Part print with two shaded views. Sizes in mm from the minimum x, y, z corner. A direction names the side the tool comes from. Round coordinates to 2 decimals unless told otherwise and drop trailing zeros. Write each loop counter-clockwise with the first axis right and the second up, starting at its lowest first coordinate (ties: lowest second). Pieces come first, ordered by that corner, then holes. Notation, with made-up numbers: (-31, -4.75) - (27, -4.75) arc R17 cw to (27, 4.25) - close; hole circle Ø7 at (-34, 63). An arc over 180 degrees is marked (long way). Answer as a JSON object with one key per item and string values. Group by question number.
Item 1: Flat gauge pin, fed straight in: pin 1 (1.5 mm diameter, centred on x = 41, z = 7.5, fed in from +Y). Where does the tip first touch, or does it go through?
Item 2: Slice it at B-B, the plane x = 22.86. List the corners of the cut face in (y, z).
Item 3: Two-plate mould, pull along X, no slides. Class the marked faces 1, 2 and 3: +X half, -X half, draft (parallel to the pull), parting line (faces both ways), or undercut.
Item 4: Which spindle directions (+Z, -Z, +X, -X, +Y, -Y) get a long thin tool onto all of the face, cutting with end or side? Do the marked faces 4 and 5. Say none if no direction does.
Item 5: Slice it at A-A, the plane z = 8.89. List the corners of the cut face in (x, y).
Item 6: Slice it at C-C, the plane y = 26. List the corners of the cut face in (x, z).
Item 7: Probe line 1 (X direction, y = 2.4, z = 8.89); line 2 (Z direction, x = 25, y = 19); line 3 (X direction, y = 35, z = 9.5). List the from-to ranges inside material, lowest first. Write a range as from..to.
Item 8: Slice it at D-D, the plane x = 10.5. List the corners of the cut face in (y, z).
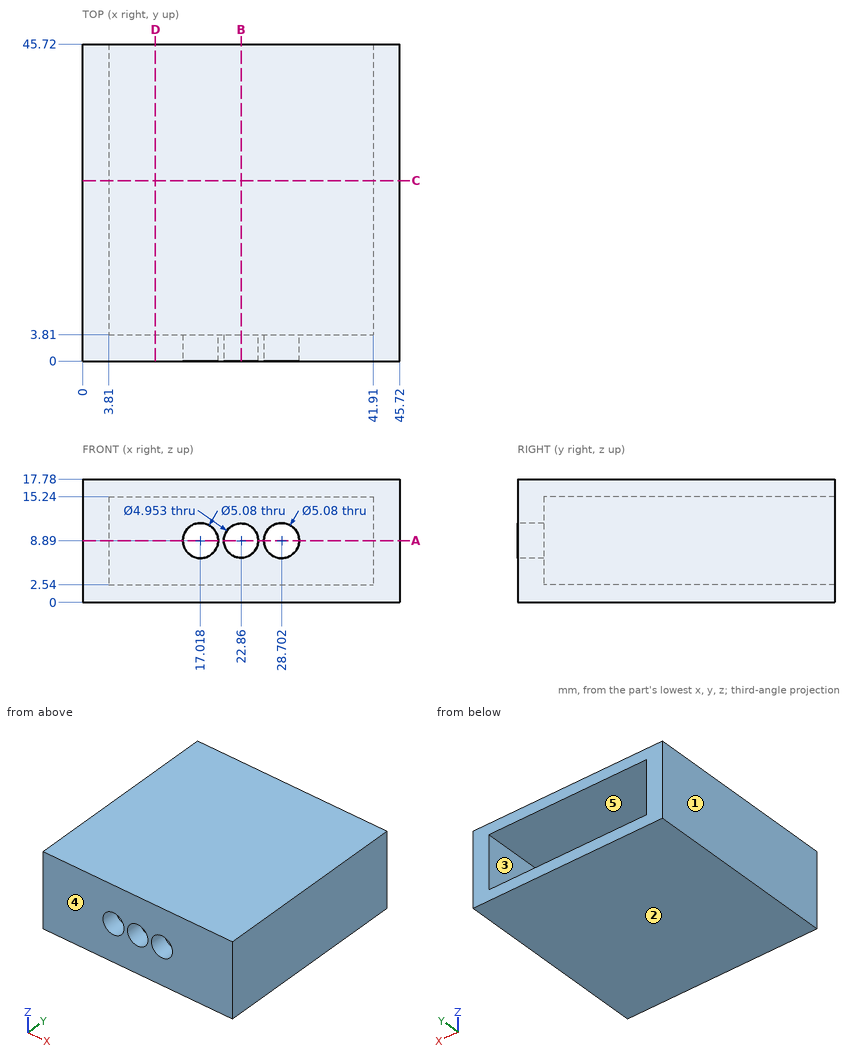
Geometry says:
{
 "1": {"pin 1": "stops at y = 3.81"},
 "2": {"outline": "(0, 0) - (45.72, 0) - (45.72, 2.54) - (3.81, 2.54) - (3.81, 6.41) - (0, 6.41) - close; (0, 11.37) - (3.81, 11.37) - (3.81, 15.24) - (45.72, 15.24) - (45.72, 17.78) - (0, 17.78) - close"},
 "3": {"face 1": "-X half", "face 2": "draft", "face 3": "undercut"},
 "4": {"face 4": "+Z, -Z, +X, -X, -Y", "face 5": "+Y"},
 "5": {"outline": "(0, 0) - (14.48, 0) - (14.48, 3.81) - (3.81, 3.81) - (3.81, 45.72) - (0, 45.72) - close; (19.56, 0) - (20.38, 0) - (20.38, 3.81) - (19.56, 3.81) - close; (25.34, 0) - (26.16, 0) - (26.16, 3.81) - (25.34, 3.81) - close; (31.24, 0) - (45.72, 0) - (45.72, 45.72) - (41.91, 45.72) - (41.91, 3.81) - (31.24, 3.81) - close"},
 "6": {"outline": "(0, 0) - (45.72, 0) - (45.72, 17.78) - (0, 17.78) - close; hole (3.81, 2.54) - (41.91, 2.54) - (41.91, 15.24) - (3.81, 15.24) - close"},
 "7": {"line 1": "x = 0..14.48, 19.56..20.38, 25.34..26.16, 31.24..45.72", "line 2": "z = 0..2.54, 15.24..17.78", "line 3": "x = 0..3.81, 41.91..45.72"},
 "8": {"outline": "(0, 0) - (45.72, 0) - (45.72, 2.54) - (3.81, 2.54) - (3.81, 15.24) - (45.72, 15.24) - (45.72, 17.78) - (0, 17.78) - close"}
}
